Geometry: final body of the model. Coordinates: model frame, mm. A direction names the side the tool comes from. Round coordinates to 2 decimals unless told otherwise and drop trailing zeros. Write each loop counter-clockwise with the first axis right and the second up, starting at its lowest first coordinate (ties: lowest second). Pieces come first, ordered by that corner, then holes. Notation, with made-up numbers: M 36.25,85.25 L 53.25,85.25 A14 ccw 53.25,98.25 Z; hole C 69.5,-20 d10. An arc over 180 degrees is marked long. Answer as CSV lines item,"result". Start each with the question number.
Q1. Section query A-A on x = -150. Output: boundary loops of the cut face in (y, z), and give its area (3 significant figures).
Q2. Mould query, pull axis X, two halves, no side actions, for faces 1 (the flat face through (-71, 0, -136)), 2 (the cylindrical face through (-151.87, 4.93, -159.98)), 3 (the flat face through (300, 8, 3)). Classes: pulls with the +X half, pulls with the -X half, needs draft (parallel to the pull), parting line crosses it, or undercut.
Q3. Section query D-D on x = 202. Output: boundary loops of the cut face in (y, z), and give its area (3 significant figures).
Q4. First-contact query: pin 1 (8 mm diameter, centred on x = 285, z = 183.68, fed in from -Y); pin 2 (4 mm diameter, centred on x = 0, z = -183.68, fed in from -Y); pin 3 (3 mm diameter, centred on x = -285, z = -183.68, fed in from -Y). Flat tips, straight axial feed; report the tip coordinate or a pass-through.
Q5. Section query C-C on y = 4.5. Give the number of separate pieces and of enclosed holes in the cut face, and give its area (3 significant figures).
Q6. Ray query, probe 1 along X at (y, z) = (9.25, -183.68); probe 2 along Z at (x, y) = (285, 10); probe 3 along X at (y, z) = (5.5, 31.5). Return the intervals inside material, ascending.
Q7. Reachability of faces 4 (the flat face through (-26, 10, 1)), 5 (the flat face through (-71, 20, -3)), 6 (the cylindrical face through (51.65, 14.93, 149.98)), 7 (the flat face through (-300, 8, 3)), 8 (the flat face through (-4, 15, -200)) from +Z, -Z, +X, -X, +Y, -Y: full face, straight path, thin tool, end or side. Return the list, or none.
Q8. Section query B-B on z = 138.5. Output: boundary loops of the cut face in (x, y), and give its area (3 significant figures).
```python
from build123d import *

# Parameters (mm, degrees)
SKETCH_1_W             = 600
SKETCH_1_H             = 400
EXTRUDE_1_DEPTH        = 30
SKETCH_2_W             = 600
SKETCH_2_H             = 388.6
CUT_EXTRUDE_1_DEPTH    = 10
SKETCH_3_W             = 50
SKETCH_3_H             = 350
CUT_EXTRUDE_2_DEPTH    = 10
SKETCH_4_W             = 40
SKETCH_4_H             = 340
CUT_EXTRUDE_3_DEPTH    = 10
HOLE_WIZARD_M6_1_D     = 5
HOLE_WIZARD_M6_1_DEPTH = 14
HOLE_WIZARD_M6_1_TIP   = 1.502151548


with BuildPart() as part:
    # 草图1 → 凸台-拉伸1 (new body)
    with BuildSketch(Plane(origin=(0, 0, 0), x_dir=(1, 0, 0), z_dir=(0, 1, 0))):
        Rectangle(SKETCH_1_W, SKETCH_1_H)
    extrude(amount=EXTRUDE_1_DEPTH)

    # 草图2 → 切除-拉伸1 (cut)
    with BuildSketch(Plane(origin=(0, 30, 0), x_dir=(1, 0, 0), z_dir=(0, 1, 0))):
        Rectangle(SKETCH_2_W, SKETCH_2_H)
    extrude(amount=-CUT_EXTRUDE_1_DEPTH, mode=Mode.SUBTRACT)

    # 草图3 → 切除-拉伸2 (cut)
    with BuildSketch(Plane.XZ):
        with Locations((200, 0)):
            Rectangle(SKETCH_3_W, SKETCH_3_H)
        with BuildLine():
            Line((-235, 75), (-235, -75))
            ThreePointArc((-235, -75), (-150, -160), (-65, -75))
            Line((-65, -75), (-65, 75))
            ThreePointArc((-65, 75), (-150, 160), (-235, 75))
        make_face()
        with BuildLine():
            Line((-35, 75), (-35, -75))
            ThreePointArc((-35, -75), (50, -160), (135, -75))
            Line((135, -75), (135, 75))
            ThreePointArc((135, 75), (50, 160), (-35, 75))
        make_face()
    extrude(amount=-CUT_EXTRUDE_2_DEPTH, mode=Mode.SUBTRACT)

    # 草图4 → 切除-拉伸3 (cut)
    with BuildSketch(Plane.XZ.offset(-10)):
        with Locations((200, 0)):
            Rectangle(SKETCH_4_W, SKETCH_4_H)
        with BuildLine():
            Line((-225, 75), (-225, -75))
            ThreePointArc((-225, -75), (-150, -150), (-75, -75))
            Line((-75, -75), (-75, 75))
            ThreePointArc((-75, 75), (-150, 150), (-225, 75))
        make_face()
        with BuildLine():
            Line((-25, 75), (-25, -75))
            ThreePointArc((-25, -75), (50, -150), (125, -75))
            Line((125, -75), (125, 75))
            ThreePointArc((125, 75), (50, 150), (-25, 75))
        make_face()
    extrude(amount=-CUT_EXTRUDE_3_DEPTH, mode=Mode.SUBTRACT)

    # M6 螺纹孔1
    with Locations(Plane(origin=(0, 0, 0), x_dir=(-1, 0, 0), z_dir=(0, -1, 0))):
        with Locations((285, -183.68), (0, -183.68), (-285, -183.68), (-285, 183.68), (0, 183.68), (285, 183.68)):
            Hole(HOLE_WIZARD_M6_1_D / 2, depth=HOLE_WIZARD_M6_1_DEPTH)
            with Locations((0, 0, -(HOLE_WIZARD_M6_1_DEPTH + HOLE_WIZARD_M6_1_TIP / 2))):  # 118° drill point
                Cone(0, HOLE_WIZARD_M6_1_D / 2, HOLE_WIZARD_M6_1_TIP, mode=Mode.SUBTRACT)


solid = part.part
```
Entries:
1,outline,"M 0,-200 L 30,-200 L 30,-194.3 L 20,-194.3 L 20,-150 L 10,-150 L 10,-160 L 0,-160 Z; M 0,160 L 10,160 L 10,150 L 20,150 L 20,194.3 L 30,194.3 L 30,200 L 0,200 Z"
1,area,"1,910 mm^2"
2,face 1,"needs draft"
2,face 2,"undercut"
2,face 3,"pulls with the +X half"
3,outline,"M 0,-200 L 30,-200 L 30,-194.3 L 20,-194.3 L 20,-170 L 10,-170 L 10,-175 L 0,-175 Z; M 0,175 L 10,175 L 10,170 L 20,170 L 20,194.3 L 30,194.3 L 30,200 L 0,200 Z"
3,area,"1,210 mm^2"
4,pin 1,"stops at y = 0"
4,pin 2,"stops at y = 14.3"
4,pin 3,"stops at y = 14.6"
5,separate pieces,"1"
5,enclosed holes,"9"
5,area,"126,000 mm^2"
6,probe 1,"x = -300 to -287.5, -282.5 to -2.5, 2.5 to 282.5, 287.5 to 300"
6,probe 2,"z = -200 to -186.18, -181.18 to 181.18, 186.18 to 200"
6,probe 3,"x = -300 to -235, -65 to -35, 135 to 175, 225 to 300"
7,face 4,"-Y"
7,face 5,"+X, -X, +Y"
7,face 6,"+Y, -Y"
7,face 7,"+Z, -Z, -X, +Y, -Y"
7,face 8,"-Z, +X, -X, +Y, -Y"
8,outline,"M -300,0 L -206.5,0 L -206.5,10 L -189.91,10 L -189.91,20 L -300,20 Z; M -110.09,10 L -93.5,10 L -93.5,0 L -6.5,0 L -6.5,10 L 10.09,10 L 10.09,20 L -110.09,20 Z; M 89.91,10 L 106.5,10 L 106.5,0 L 175,0 L 175,10 L 180,10 L 180,20 L 89.91,20 Z; M 220,10 L 225,10 L 225,0 L 300,0 L 300,20 L 220,20 Z"
8,area,"7,240 mm^2"
